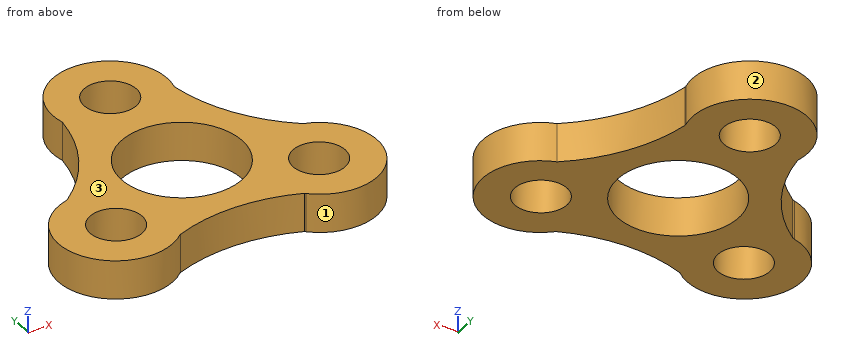
```python
from build123d import *

# Parameters (mm, degrees)
F0_R     = 10.92
F0_R_2   = 4.7275
F1_DEPTH = 7


with BuildPart() as f1:
    # F0 (on Top) → F1 (new body)
    with BuildSketch(Plane.XY):
        Circle(F0_R)
        with BuildLine():
            Line((11.151573, -18.07834), (11.331202, -18.274194))
            ThreePointArc((11.331202, -18.274194), (27.437316, -15.933644), (21.448669, -0.800199))
            ThreePointArc((21.448669, -0.800199), (13.899631, 7.78037), (10.100635, 18.559135))
            Line((10.100635, 18.559135), (10.160315, 18.950206))
            ThreePointArc((10.160315, 18.950206), (0.080283, 31.728235), (-10.031342, 18.975192))
            ThreePointArc((-10.031342, 18.975192), (-13.660086, 8.19612), (-21.035123, -0.462112))
            Line((-21.035123, -0.462112), (-21.491517, -0.676012))
            ThreePointArc((-21.491517, -0.676012), (-27.517599, -15.79459), (-11.417327, -18.174993))
            ThreePointArc((-11.417327, -18.174993), (-0.142296, -15.92724), (11.151573, -18.07834))
        make_face()
        with Locations((-18.405074, -10.591076)):
            Circle(F0_R_2, mode=Mode.SUBTRACT)
        with Locations((18.374678, -10.643723)):
            Circle(F0_R_2, mode=Mode.SUBTRACT)
        Circle(F0_R, mode=Mode.SUBTRACT)
        with Locations((0.030396, 21.234799)):
            Circle(F0_R_2, mode=Mode.SUBTRACT)
    extrude(amount=F1_DEPTH)


solid = f1.part
```
Could you check a few things on this model? Use its own coordinates, in mm. Face numbers are marked on the shaded views. Round coordinates to 2 decimals unless told otherwise and drop trailing zeros. Loops run counter-clockwise (first coordinate to the right, second up) from the corner with the lowest first, then second, coordinate; pieces in that order, holes last. Notation, with made-up numbers: (-34, 58.25) - (-21, 58.25) arc R18 cw to (-21, 69.25) - close; hole circle Ø5 at (68.5, 62). An arc over 180 degrees is marked (long way). Answer in a Markdown table with one row per item. Add a question column.
(1) If we section it at C-C (x = 0): Please give me the cut outline in (y, z).
(2) If we section it at B-B (x = -15): Please give me the cut outline in (y, z).
(3) If we section it at A-A (y = -17): Please give me the cut outline in (x, z).
(4) If we section it at D-D (z = 0.75): State how many separate pieces and enclosed holes the cut face has, plus the area to 3 significant figures.
(5) I need wall thicknesses on line 1 along Y through (x, z) = (0, 2.5); line 2 along Y through (x, z) = (-3.5, 5.5); line 3 along X through (y, z) = (-9.5, 4.5). Which ranges of each line are inside material? Lowest first, please.
(6) If we mould it in two halves opening along X, with no side actions, what happens to the marked faces 1, 2 and 3? For each: pulls with the +X half, pulls with the -X half, needs draft (parallel to the pull), parting line crosses it, or undercut.
(7) I'm going to push flat-ended pins straight in: pin 1 (5.5 mm diameter, centred on x = 0.03, y = 21.23, fed in from -Z); pin 2 (3 mm diameter, centred on x = 16, z = 6, fed in from -Y). Where does each tip first touch, or does it pass through?
Model answer:
| question | item | result |
|---|---|---|
| 1 | outline | (-15.93, 0) - (-10.92, 0) - (-10.92, 7) - (-15.93, 7) - close; (10.92, 0) - (16.51, 0) - (16.51, 7) - (10.92, 7) - close; (25.96, 0) - (31.73, 0) - (31.73, 7) - (25.96, 7) - close |
| 2 | outline | (-20.38, 0) - (-13.87, 0) - (-13.87, 7) - (-20.38, 7) - close; (-7.31, 0) - (6.05, 0) - (6.05, 7) - (-7.31, 7) - close |
| 3 | outline | (-26.71, 0) - (-7.97, 0) - (-7.97, 7) - (-26.71, 7) - close; (7.94, 0) - (26.73, 0) - (26.73, 7) - (7.94, 7) - close |
| 4 | separate pieces | 1 |
| 4 | enclosed holes | 4 |
| 4 | area | 1,160 mm² |
| 5 | line 1 | y = -15.93 to -10.92, 10.92 to 16.51, 25.96 to 31.73 |
| 5 | line 2 | y = -16.13 to -10.34, 10.34 to 18.09, 24.38 to 31.1 |
| 5 | line 3 | x = -28.84 to -23, -13.81 to -5.38, 5.38 to 13.79, 22.96 to 28.76 |
| 6 | face 1 | undercut |
| 6 | face 2 | parting line crosses it |
| 6 | face 3 | needs draft |
| 7 | pin 1 | passes through |
| 7 | pin 2 | stops at y = -21.07 |
